from build123d import *
from build123d import SkipClean  # not in build123d's __all__

# Parameters (mm, degrees)
F1_DEPTH  = 4
F2_R      = 3
F3_R      = 1
F4_R      = 0.5
F6_DEPTH  = 25
F8_DEPTH  = 2.8
F9_R      = 0.75
F10_W     = 9.5
F10_H     = 9.4
F10_H_2   = 5.1
F11_DEPTH = 1.9
F12_R     = 3.5
F13_R     = 1.325
F14_DEPTH = 5
F15_R     = 0.7


# Not quite as in the source:
# - after a boolean that leaves OpenCascade's solid faulty, fix() repairs it


with BuildPart() as f1:
    # F0 (on Front) → F1 (new body)
    with BuildSketch(Plane.XZ):
        Polygon((0, 11.3), (0, 0), (-37.3, 0), (-37.3, -4.37), (-6.42, -35.25), (8.2981568685, -22.9), (38.5981568685, -22.9), (18.8527776623, 11.3), align=None)
    extrude(amount=F1_DEPTH)

    # F2
    f2_edges = [f1.edges().sort_by_distance(p)[0] for p in [
        (-37.3, -2, -4.37),
        (18.852778, -2, 11.3),
    ]]
    fillet(f2_edges, radius=F2_R)

    # F3
    f3_edges = [f1.edges().sort_by_distance(p)[0] for p in [
        (38.598157, -2, -22.9),
        (-6.42, -2, -35.25),
    ]]
    fillet(f3_edges, radius=F3_R)

    # F4
    f4_edges = [f1.edges().sort_by_distance(p)[0] for p in [
        (8.298157, -2, -22.9),
        (0, -2, 0),
        (0, -2, 11.3),
        (-37.3, -2, 0),
    ]]
    fillet(f4_edges, radius=F4_R)

    # F5 (on face) → F6 (cut)
    with BuildSketch(Plane.XZ.offset(4)):
        with BuildLine():
            Line((13.3, -4.33), (-7.5, -4.33))
            ThreePointArc((-7.5, -4.33), (2.9, -16.93), (13.3, -4.33))
        make_face()
    extrude(amount=-F6_DEPTH, mode=Mode.SUBTRACT)

    # F7 (on face) → F8 (join)
    with BuildSketch(Plane.XZ.offset(4)):
        with BuildLine():
            Line((15.15, -2.33), (-9.35, -2.33))
            Line((-9.35, -2.33), (-9.35, -6.44))
            Line((-9.35, -6.44), (-7.6915717466, -6.44))
            ThreePointArc((-7.6915717466, -6.44), (-7.6486750873, -5.3801980668), (-7.5, -4.33))
            Line((-7.5, -4.33), (13.3, -4.33))
            ThreePointArc((13.3, -4.33), (13.4486750873, -5.3801980668), (13.4915717466, -6.44))
            Line((13.4915717466, -6.44), (15.15, -6.44))
            Line((15.15, -6.44), (15.15, -2.33))
        make_face()
    with SkipClean():  # cleaning this boolean's faces spoils the solid; the shape is the same uncleaned
        extrude(amount=F8_DEPTH)

    # F9
    f9_edges = [f1.edges().sort_by_distance(p)[0] for p in [
        (-9.35, -5.4, -2.33),
        (15.15, -5.4, -2.33),
    ]]
    fillet(f9_edges, radius=F9_R)

    # F10 (on face) → F11 (join)
    with BuildSketch(Plane(origin=(0, 0, 0), x_dir=(-1, 0, 0), z_dir=(0, 1, 0))):
        with Locations((21.49, 4.7)):
            Rectangle(F10_W, F10_H)
        with Locations((21.49, -2.55)):
            Rectangle(F10_W, F10_H_2)
        Polygon((17.8186578158, -23.8513421842), (24.5361722371, -17.1338277629), (20.929927653, -13.5275831789), (14.2124132317, -20.2450976002), align=None)
        Polygon((31.1829759802, -23.7806315061), (24.5361722371, -17.1338277629), (17.8186578158, -23.8513421842), (24.4654615589, -30.4981459274), align=None)
    extrude(amount=F11_DEPTH)

    add(f1.part.fix(), mode=Mode.REPLACE)

    # F12
    f12_edges = [f1.edges().sort_by_distance(p)[0] for p in [
        (-24.465462, 0.95, -30.498146),
        (-31.182976, 0.95, -23.780632),
        (-14.212413, 0.95, -20.245098),
        (-20.929928, 0.95, -13.527583),
        (-26.24, 0.95, 9.4),
        (-16.74, 0.95, 9.4),
        (-26.24, 0.95, -5.1),
        (-16.74, 0.95, -5.1),
    ]]
    fillet(f12_edges, radius=F12_R)

    # F13 (on face) → F14 (join)
    with BuildSketch(Plane(origin=(0, 0, 0), x_dir=(-1, 0, 0), z_dir=(0, 1, 0))):
        with Locations((-22.6430821795, -6.115)):
            Circle(F13_R)
    extrude(amount=F14_DEPTH)

    # F15
    f15_edges = [f1.edges().sort_by_distance(p)[0] for p in [
        (23.968082, 5, -6.115),
    ]]
    fillet(f15_edges, radius=F15_R)


solid = f1.part
Source: CAD feature listing. Evaluate the final solid. Frame: model axes, mm. A direction names the side the tool comes from. Coordinates: 2 decimals unless noted, no trailing zeros. Order: outer loops, then holes, each group sorted by start corner. A loop starts at its lowest first (then second) coordinate and runs counter-clockwise, first axis right, second up. Notation, with made-up numbers: M 51,11.5 L 78,11.5 A20 ccw 78,30.5 Z; hole C -19,4 d3. An arc over 180 degrees is marked long. Write each question's results on one line, items separated by ' | '. Start each with the question number.
Item 1: Set-up query: faces 1 (the face through (-17.584, 0.937, -16.874)), 2 (the face through (-21.95, -1.97, -19.72)), 3 (the face through (-26.24, 1, 2)), 4 (the face through (21.42, 2.12, -6.62)), 5 (the face through (14, -5, -6.44)). Return all of +Z, -Z, +X, -X, +Y, -Y with unobstructed straight access to the full face (end or side cutting, diameter ignored); none if empty.
Item 2: First-contact query: pin 1 Ø1 at (x, y) = (-22, 0.5) entering from -Z; pin 2 Ø3 at (y, z) = (-6, -4.5) entering from -X; pin 3 Ø0.8 at (x, y) = (14.5, -6) entering from -Z; pin 4 Ø2 at (x, z) = (-3.5, -12) entering from -Y. Flat tips, straight axial feed; report the tip coordinate or a pass-through.
Item 3: Draft query along Z for faces 6 (the face through (0, -4, -17)), 7 (the face through (-15.662, 0.963, -20.284)), 8 (the face through (-21, 1, -5.1)). Return one class per face: pulls with the +Z half, pulls with the -Z half, needs draft (parallel to the pull), parting line crosses it, or undercut.
Item 4: Cut plane A-A (x = 2.9). Return loops of the section in (y, z), and give its area (3 significant figures).
Item 5: Line query: probe 1 along Y at (x, z) = (-22, -15); probe 2 along Z at (x, y) = (6, -6); probe 3 along X at (y, z) = (1.25, 6). Output: solid intervals per line, ascending.
Item 6: Cut plane C-C (x = -13). Return loops of the section in (y, z), and give its area (3 significant figures).
Item 7: Cut plane B-B (y = -5.75). Return loops of the section in (x, z).
Checked values:
1) face 1: +X, +Y | face 2: -Z, -X, -Y | face 3: +Z, -X, +Y | face 4: +Y | face 5: -Z, +X, -X, -Y
2) pin 1: stops at z = -28.44 | pin 2: stops at x = -9.35 | pin 3: stops at z = -6.44 | pin 4: passes through
3) face 6: needs draft | face 7: parting line crosses it | face 8: undercut
4) outline: M -6.8,-4.33 L 0,-4.33 L 0,11.3 L -4,11.3 L -4,-2.33 L -6.8,-2.33 Z; M -4,-27.43 L 0,-27.43 L 0,-16.93 L -4,-16.93 Z | area: 110 mm2
5) probe 1: y = -4 to 0 | probe 2: z = -4.33 to -2.33 | probe 3: x = -26.24 to -16.74
6) outline: M -4,-28.67 L 0,-28.67 L 0,0 L -4,0 Z | area: 115 mm2
7) outline: M -9.35,-6.44 L -7.69,-6.44 A10.59 cw -7.5,-4.33 L 13.3,-4.33 A10.59 cw 13.49,-6.44 L 15.15,-6.44 L 15.15,-3.08 A0.75 ccw 14.4,-2.33 L -8.6,-2.33 A0.75 ccw -9.35,-3.08 Z
